The model under review builds one solid part; all positions refer to its coordinate system, in mm. A direction names the side the tool comes from. Coordinates: 2 decimals unless noted, no trailing zeros. Order: outer loops, then holes, each group sorted by start corner. A loop starts at its lowest first (then second) coordinate and runs counter-clockwise, first axis right, second up. Notation, with made-up numbers: M 79,77 L 88,77 A10 cw 88,93 Z; hole C -33,23.5 d11. An arc over 180 degrees is marked long. Answer in a Markdown table with one row per item.
from build123d import *

# Parameters (mm, degrees)
SKETCH_1_W          = 1000
SKETCH_1_H          = 1200
EXTRUDE_1_DEPTH     = 75
CUT_EXTRUDE_1_REACH = 1304.162
SKETCH_2_W          = 340
SKETCH_2_H          = 125
SKETCH_3_W          = 320
SKETCH_3_H          = 90
CUT_EXTRUDE_2_DEPTH = 1169.599589252


with BuildPart() as part:
    # 草图1 → 凸台-拉伸1 (new, symmetric)
    with BuildSketch(Plane(origin=(0, 0, 0), x_dir=(1, 0, 0), z_dir=(0, 1, 0))):
        Rectangle(SKETCH_1_W, SKETCH_1_H)
    extrude(amount=EXTRUDE_1_DEPTH, both=True)

    # 草图2 → 切除-拉伸1 (cut, up to next)
    with BuildSketch(Plane.XY.offset(600), mode=Mode.PRIVATE) as cut_extrude_1_sk1:
        with Locations((-230, -12.5)):
            Rectangle(SKETCH_2_W, SKETCH_2_H)
    cut_extrude_1_tool1 = extrude(cut_extrude_1_sk1.sketch, amount=-CUT_EXTRUDE_1_REACH, mode=Mode.PRIVATE) & part.part
    # 草图2 → 切除-拉伸1 (cut, up to next)
    with BuildSketch(Plane.XY.offset(600), mode=Mode.PRIVATE) as cut_extrude_1_sk2:
        with Locations((230, -12.5)):
            Rectangle(SKETCH_2_W, SKETCH_2_H)
    cut_extrude_1_tool2 = extrude(cut_extrude_1_sk2.sketch, amount=-CUT_EXTRUDE_1_REACH, mode=Mode.PRIVATE) & part.part
    add(cut_extrude_1_tool1.solids().sort_by_distance((-230, -12.5, 600))[0], mode=Mode.SUBTRACT)
    add(cut_extrude_1_tool2.solids().sort_by_distance((230, -12.5, 600))[0], mode=Mode.SUBTRACT)

    # 草图3 → 切除-拉伸2 (cut, through all)
    with BuildSketch(Plane.ZY.offset(500)):
        with Locations((260, 5)):
            Rectangle(SKETCH_3_W, SKETCH_3_H)
        with Locations((-260, 5)):
            Rectangle(SKETCH_3_W, SKETCH_3_H)
    extrude(amount=-CUT_EXTRUDE_2_DEPTH, mode=Mode.SUBTRACT)


solid = part.part
(1) Take a section at A-A (z = 325). Write out the cut boundary in (x, y).
Report:
| item | result |
|---|---|
| outline | M -500,-75 L -400,-75 L -400,-40 L -500,-40 Z; M -500,50 L 500,50 L 500,75 L -500,75 Z; M -60,-75 L 60,-75 L 60,-40 L -60,-40 Z; M 400,-75 L 500,-75 L 500,-40 L 400,-40 Z |
(2) Take a section at B-B (x = -29.5). Write out the cut boundary in (y, z), then the cut area to 3 significant figures.
Report:
| item | result |
|---|---|
| outline | M -75,-600 L 75,-600 L 75,600 L -75,600 Z; hole M -40,-420 L 50,-420 L 50,-100 L -40,-100 Z; hole M -40,100 L 50,100 L 50,420 L -40,420 Z |
| area | 122,000 mm^2 |
(3) To check wall thickness, follow line 1 (Z direction, x = 437, y = -25); line 2 (X direction, y = -63, z = -205.5); line 3 (Y direction, x = 55, z = 297). State the ranges of each line that lie inside material, in increasing order. Write a range as [from, to].
Report:
| item | result |
|---|---|
| line 1 | [-600, -420], [-100, 100], [420, 600] |
| line 2 | [-500, -400], [-60, 60], [400, 500] |
| line 3 | [-75, -40], [50, 75] |
(4) The part is to be moulded in two halves that separate along Y. For faces 4 (the flat face through (449, 4, 420)), 5 (the flat face through (-400, -27, 8)), 6 (the flat face through (449, 4, 100)), say which applies: +Y half, -Y half, draft (parallel to the pull), parting line (faces both ways), or undercut.
Report:
| item | result |
|---|---|
| face 4 | undercut |
| face 5 | draft |
| face 6 | undercut |
(5) Take a section at C-C (y = -25). State how many separate pieces and enclosed holes the cut face has, then the cut area to 3 significant figures.
Report:
| item | result |
|---|---|
| separate pieces | 9 |
| enclosed holes | 0 |
| area | 179,000 mm^2 |
(6) Take a section at D-D (z = -518.5). Write out the cut boundary in (x, y).
Report:
| item | result |
|---|---|
| outline | M -500,-75 L -400,-75 L -400,50 L -60,50 L -60,-75 L 60,-75 L 60,50 L 400,50 L 400,-75 L 500,-75 L 500,75 L -500,75 Z |
(7) Machinability: for faces 1 (the flat face through (60, -27, 8)), 2 (the flat face through (-451, 4, 420)), 3 (the flat face through (104, 50, -8)), which of the approach directions +Z, -Z, +X, -X, +Y, -Y give a long, thin tool a straight path to every point of the face, cutting with its end or side? Answer none if there is none.
Report:
| item | result |
|---|---|
| face 1 | +Z, -Z, -Y |
| face 2 | +X, -X |
| face 3 | none |
